Here's how the part is built. I have some questions about the finished solid (model axes, mm). A direction names the side the tool comes from. Coordinates: 2 decimals unless noted, no trailing zeros. Loops run counter-clockwise (first coordinate to the right, second up) from the corner with the lowest first, then second, coordinate; pieces in that order, holes last.
from build123d import *

# Parameters (mm, degrees)
SKETCH_1_R               = 11
EXTRUDE_1_DEPTH          = 180
SKETCH_2_R               = 9
EXTRUDE_2_DEPTH          = 5
CUT_EXTRUDE_1_DEPTH      = 186.652901943
CUT_EXTRUDE_1_DEPTH_BACK = 186.652901943
SKETCH_3_R               = 7


with BuildPart() as part:
    # 草图1 → 凸台-拉伸1 (new body)
    with BuildSketch(Plane.XY):
        with Locations(Location((0, 0, 0), (0, 0, 180))):
            Circle(SKETCH_1_R)
    extrude(amount=EXTRUDE_1_DEPTH)

    # 草图2 → 凸台-拉伸2 (add)
    with BuildSketch(Plane.XY.offset(180)):
        Circle(SKETCH_2_R)
    extrude(amount=EXTRUDE_2_DEPTH)

    # 草图3 → 切除-拉伸1 (cut, two sides: drawn at the far end of the back side and taken through both)
    with BuildSketch(Plane(origin=(0, 0, 0), x_dir=(-1, 0, 0), z_dir=(0, 0, -1)).offset(-CUT_EXTRUDE_1_DEPTH_BACK)):
        Circle(SKETCH_3_R)
    extrude(amount=CUT_EXTRUDE_1_DEPTH + CUT_EXTRUDE_1_DEPTH_BACK, mode=Mode.SUBTRACT)


solid = part.part
Q1. Please list where these lines run through material, in increasing order: probe 1 along Y at (x, z) = (0, 70); probe 2 along Z at (x, y) = (7.25, 6.75); probe 3 along X at (y, z) = (-3.5, 21.5).
Q2. Will these pins go through, and if not, where does the flat tip stop? P1, Ø3, axis at x = -6.5, z = 122, coming from the +Y side; P2, Ø1, axis at x = -7.5, z = 76, coming from the +Y side.
Q3. We'd pull the mould along Y, two halves only. Please class faces 3 (the flat face through (-7.2, -0.2, 0)), 4 (the cylindrical face through (2.38, 10.74, 88.74)), 5 (the cylindrical face through (-6.466, -2.681, 93.795)): pulls with the +Y half, pulls with the -Y half, needs draft (parallel to the pull), parting line crosses it, or undercut.
Q4. Suppose I cut it at B-B on y = 2.5. Write out the boundary of the cut face in (x, z).
Q5. For faces 1 (the cylindrical face through (-1.172, 8.923, 182.465)), 2 (the flat face through (0, -7.3, 185)), which set-ups out of +Z, -Z, +X, -X, +Y, -Y let a thin tool reach every point of the face, with its end or its side?
Q6. Suppose I cut it at C-C on z = 15.5. Write out the boundary of the cut face in (x, y), and give its area (3 significant figures).
Q7. Suppose I cut it at A-A on x = 0. Write out the boundary of the cut face in (y, z).
Check values:
1. probe 1: y = -11 to -7, 7 to 11
1. probe 2: z = 0 to 180
1. probe 3: x = -10.43 to -6.06, 6.06 to 10.43
2. P1: stops at y = 9.8
2. P2: stops at y = 8.49
3. face 3: needs draft
3. face 4: parting line crosses it
3. face 5: undercut
4. outline: (-10.71, 0) - (-6.54, 0) - (-6.54, 185) - (-8.65, 185) - (-8.65, 180) - (-10.71, 180) - close; (6.54, 0) - (10.71, 0) - (10.71, 180) - (8.65, 180) - (8.65, 185) - (6.54, 185) - close
5. face 1: +Z
5. face 2: +Z, +X, -X, +Y, -Y
6. outline: circle Ø22 at (0, 0); hole circle Ø14 at (0, 0)
6. area: 226 mm2
7. outline: (-11, 0) - (-7, 0) - (-7, 185) - (-9, 185) - (-9, 180) - (-11, 180) - close; (7, 0) - (11, 0) - (11, 180) - (9, 180) - (9, 185) - (7, 185) - close
